```python
from build123d import *

# Parameters (mm, degrees)
SKETCH1_W           = 98
SKETCH1_H           = 66
SKETCH1_R           = 1.25
BOSS_EXTRUDE1_DEPTH = 2
SKETCH1_3_R         = 1.25
BOSS_EXTRUDE2_DEPTH = 32
SKETCH2_W           = 98
SKETCH2_H           = 66
BOSS_EXTRUDE3_DEPTH = 25
CUT_EXTRUDE1_DEPTH  = 25
BOSS_EXTRUDE4_DEPTH = 95
SKETCH5_W           = 24
SKETCH5_H           = 23.3
BOSS_EXTRUDE5_DEPTH = 2
BOSS_EXTRUDE6_DEPTH = 0.3
BOSS_EXTRUDE7_DEPTH = 0.7
CUT_EXTRUDE2_DEPTH  = 2


with BuildPart() as part:
    # Sketch1 → Boss-Extrude1 (new body)
    with BuildSketch(Plane.XY):
        with Locations((44, 28)):
            Rectangle(SKETCH1_W, SKETCH1_H)
        with Locations((61.5, 3.5)):
            Circle(SKETCH1_R, mode=Mode.SUBTRACT)
        with Locations((3.5, 52.5)):
            Circle(SKETCH1_R, mode=Mode.SUBTRACT)
        with Locations((61.5, 52.5)):
            Circle(SKETCH1_R, mode=Mode.SUBTRACT)
        with Locations((3.5, 3.5)):
            Circle(SKETCH1_R, mode=Mode.SUBTRACT)
    extrude(amount=BOSS_EXTRUDE1_DEPTH)

    # Sketch1<3> → Boss-Extrude2 (add)
    with BuildSketch(Plane.XY):
        with Locations((3.5, 52.5)):
            Circle(SKETCH1_3_R)
        with Locations((61.5, 52.5)):
            Circle(SKETCH1_3_R)
        with Locations((61.5, 3.5)):
            Circle(SKETCH1_3_R)
        with Locations((3.5, 3.5)):
            Circle(SKETCH1_3_R)
    extrude(amount=BOSS_EXTRUDE2_DEPTH)

    # Sketch2 → Boss-Extrude3 (add)
    with BuildSketch(Plane(origin=(0, 0, 0), x_dir=(-1, 0, 0), z_dir=(0, 0, -1))):
        with BuildLine():
            Line((7, -5), (7, 61))
            ThreePointArc((7, 61), (6.414213562, 62.414213562), (5, 63))
            Line((5, 63), (-93, 63))
            ThreePointArc((-93, 63), (-94.414213562, 62.414213562), (-95, 61))
            Line((-95, 61), (-95, -5))
            ThreePointArc((-95, -5), (-94.414213562, -6.414213562), (-93, -7))
            Line((-93, -7), (5, -7))
            ThreePointArc((5, -7), (6.414213562, -6.414213562), (7, -5))
        make_face()
        with Locations((-44, 28)):
            Rectangle(SKETCH2_W, SKETCH2_H, mode=Mode.SUBTRACT)
    extrude(amount=-BOSS_EXTRUDE3_DEPTH)

    # Sketch3 → Cut-Extrude1 (cut)
    with BuildSketch(Plane.XZ.offset(7)):
        with BuildLine():
            Line((15.85, 10), (15.85, 2))
            Line((15.85, 2), (5.35, 2))
            Line((5.35, 2), (5.35, 10))
            ThreePointArc((5.35, 10), (5.672315931, 11.81119566), (6.599687512, 13.4))
            Line((6.599687512, 13.4), (14.600312488, 13.4))
            ThreePointArc((14.600312488, 13.4), (15.527684069, 11.81119566), (15.85, 10))
        make_face()
    extrude(amount=-CUT_EXTRUDE1_DEPTH, mode=Mode.SUBTRACT)

    # Sketch4 → Boss-Extrude4 (add)
    with BuildSketch(Plane(origin=(-5, 0, 0), x_dir=(0, 0, -1), z_dir=(1, 0, 0))):
        Polygon((-24, 84.3), (-24, 86.3), (0, 86.3), (0, 63), (-2, 63), (-2, 84.3), align=None)
    extrude(amount=BOSS_EXTRUDE4_DEPTH)

    # Sketch5 → Boss-Extrude5 (add)
    with BuildSketch(Plane(origin=(90, 0, 0), x_dir=(0, 0, -1), z_dir=(1, 0, 0))):
        with Locations((-12, 74.65)):
            Rectangle(SKETCH5_W, SKETCH5_H)
    extrude(amount=BOSS_EXTRUDE5_DEPTH)

    # Sketch6 → Boss-Extrude6 (add)
    with BuildSketch(Plane.XY.offset(24)):
        Polygon((-5, 84.3), (-5, 86.3), (92, 86.3), (92, 63), (90, 63), (90, 84.3), align=None)
    extrude(amount=BOSS_EXTRUDE6_DEPTH)

    # Sketch7 → Boss-Extrude7 (add)
    with BuildSketch(Plane(origin=(-5, 84.3, 24.3), x_dir=(1, 0, 0), z_dir=(0, 0, 1))):
        with BuildLine():
            Line((97, -21.3), (97, -9.65))
            Line((97, -9.65), (93.5, -9.65))
            ThreePointArc((93.5, -9.65), (91.303300859, -14.953300859), (86, -17.15))
            Line((86, -17.15), (0, -17.15))
            Line((0, -17.15), (0, -21.3))
            Line((0, -21.3), (97, -21.3))
        make_face()
        with BuildLine():
            Line((93.5, -9.65), (97, -9.65))
            Line((97, -9.65), (97, 2))
            Line((97, 2), (0, 2))
            Line((0, 2), (0, -2.15))
            Line((0, -2.15), (86, -2.15))
            ThreePointArc((86, -2.15), (91.303300859, -4.346699141), (93.5, -9.65))
        make_face()
    extrude(amount=BOSS_EXTRUDE7_DEPTH)

    # Sketch8 → Cut-Extrude2 (cut)
    with BuildSketch(Plane(origin=(92, 0, 0), x_dir=(0, 0, -1), z_dir=(1, 0, 0))):
        with BuildLine():
            ThreePointArc((-7.536194091, 79.62344782), (-18.12344782, 80.263805909), (-18.763805909, 69.67655218))
            Line((-18.763805909, 69.67655218), (-7.536194091, 79.62344782))
        make_face()
        with BuildLine():
            Line((-7.536194091, 79.62344782), (-18.763805909, 69.67655218))
            ThreePointArc((-18.763805909, 69.67655218), (-10.490445932, 67.637384785), (-5.65, 74.65))
            ThreePointArc((-5.65, 74.65), (-6.137384785, 77.309554068), (-7.536194091, 79.62344782))
        make_face()
    extrude(amount=-CUT_EXTRUDE2_DEPTH, mode=Mode.SUBTRACT)


solid = part.part
```
Input: part model. Units: mm. Frame: model coordinates. A direction names the side the tool comes from. Give positions to 0.01 mm unless a question says otherwise; leave off trailing zeros. Order: outer loops, then holes, each group sorted by start corner. A loop starts at its lowest first (then second) coordinate and runs counter-clockwise, first axis right, second up. Notation, with made-up numbers: M 82,-6 L 122,-6 A27 cw 122,22 Z; hole C 73.25,8 d1. An arc over 180 degrees is marked long. One line per question, with ' | ' between items.
1) Section A-A on z = 15. Output: boundary loops of the cut face in (x, y).
Filled in:
outline: M -7,-5 A2 ccw -5,-7 L 93,-7 A2 ccw 95,-5 L 95,61 A2 ccw 93,63 L 92,63 L 92,67.38 L 90,67.38 L 90,63 L -5,63 A2 ccw -7,61 Z; M -5,84.3 L 90,84.3 L 90,81.92 L 92,81.92 L 92,86.3 L -5,86.3 Z; C 3.5,3.5 d2.5; C 3.5,52.5 d2.5; C 61.5,3.5 d2.5; C 61.5,52.5 d2.5; hole M -5,-5 L 93,-5 L 93,61 L -5,61 Z
2) Contact query for flat-ended pins moving along their axis: P1, Ø3, axis at x = 76, y = 14, coming from the +Z side; P2, Ø1, axis at y = -6, z = 4.5, coming from the -X side; P3, Ø23.5, axis at x = 23.5, y = 75.5, coming from the +Z side. Output: stop coordinate, or through.
Filled in:
P1: stops at z = 2 | P2: stops at x = -6.94 | P3: stops at z = 25
3) Access query for faces 5 (the face through (43, 84.3, 13)), 6 (the face through (45, -5, 13)), 7 (the face through (92, 80, 7)). Directions: +Z, -Z, +X, -X, +Y, -Y. A direction counts if a zero-diameter tool reaches every point of the face in a straight line with its end or side. Return the directions, or none.
Filled in:
face 5: -X | face 6: +Z | face 7: +Z, -Z, +X, +Y
4) Ray query, L1, parallel to Y at x = 55, z = 8.5; L2, parallel to Y at x = 67.5, z = 24.5; L3, parallel to X at y = 46, z = 5.5. Return the intervals inside material, ascending.
Filled in:
L1: y = -7 to -5, 61 to 63, 84.3 to 86.3 | L2: y = -7 to -5, 61 to 67.15, 82.15 to 86.3 | L3: x = -7 to -5, 93 to 95
5) Section C-C on y = 43. Output: boundary loops of the cut face in (x, z), and give its area (3 significant figures).
Filled in:
outline: M -7,0 L 95,0 L 95,25 L 93,25 L 93,2 L -5,2 L -5,25 L -7,25 Z | area: 296 mm2
6) Section D-D on z = 28.5. Output: boundary loops of the cut face in (x, y).
Filled in:
outline: C 3.5,3.5 d2.5; C 3.5,52.5 d2.5; C 61.5,3.5 d2.5; C 61.5,52.5 d2.5
7) Section B-B on x = 3.5. Output: boundary loops of the cut face in (y, z), and give its area (3 significant figures).
Filled in:
outline: M -7,0 L 86.3,0 L 86.3,25 L 82.15,25 L 82.15,24.3 L 84.3,24.3 L 84.3,2 L 63,2 L 63,24.3 L 67.15,24.3 L 67.15,25 L 61,25 L 61,2 L 53.75,2 L 53.75,32 L 51.25,32 L 51.25,2 L 4.75,2 L 4.75,32 L 2.25,32 L 2.25,2 L -5,2 L -5,25 L -7,25 Z | area: 479 mm2
8) Draft query along X for faces 1 (the face through (61, 53, 32)), 2 (the face through (3.34, 53.74, 16.79)), 3 (the face through (-7, 28, 12)), 4 (the face through (62.69, 52.88, 16.79)). Return one class per face: pulls with the +X half, pulls with the -X half, needs draft (parallel to the pull), parting line crosses it, or undercut.
Filled in:
face 1: needs draft | face 2: undercut | face 3: pulls with the -X half | face 4: undercut
